Part model, mm, in its own coordinate system. A direction names the side the tool comes from. Round coordinates to 2 decimals unless told otherwise and drop trailing zeros. Loops run counter-clockwise (first coordinate to the right, second up) from the corner with the lowest first, then second, coordinate; pieces in that order, holes last. Notation, with made-up numbers: (2.25, 22) -> (53.25, 22) arc R14 ccw to (53.25, 36) -> close; hole circle Ø3 at (-27.75, 45). An arc over 180 degrees is marked (long way). Use a Markdown table: item, result. Add a question column.
Item 1: Which spindle directions (+Z, -Z, +X, -X, +Y, -Y) get a long thin tool onto all of the face, cutting with end or side? Do faces 1 (the face through (0, -12.5, 15)), 2 (the face through (-14.715, 0.231, 29.699)). Say none if no direction does.
Item 2: Cut at A-A, the plane y = 9. List the corners of the cut face in (x, z).
Item 3: Cut at C-C, the plane x = 0. List the corners of the cut face in (y, z), plus the area to 3 significant figures.
Item 4: Cut at B-B, the plane z = 15. List the corners of the cut face in (x, y).
Item 5: Two-plate mould, pull along X, no slides. Class faces 3 (the face through (-14.715, 17.199, 15.196)), 4 (the face through (1.5, 2.7, 19.77)), 5 (the face through (0.196, -17.215, 29.699)): pulls with the +X half, pulls with the -X half, needs draft (parallel to the pull), parting line crosses it, or undercut.
Item 6: Probe line 1 (X direction, y = 1, z = 15); line 2 (X direction, y = -6, z = 12); line 3 (Z direction, x = -0.75, y = 11). List the from-to ranges inside material, lowest first. Write a range as [from, to].
```python
from build123d import *

# Parameters (mm, degrees)
SKETCH1_W           = 30
SKETCH1_H           = 35
BOSS_EXTRUDE1_DEPTH = 30
SKETCH2_R           = 5
CUT_EXTRUDE1_DEPTH  = 30
FILLET2_R           = 1


with BuildPart() as part:
    # Sketch1 → Boss-Extrude1 (new body)
    with BuildSketch(Plane.XY):
        Rectangle(SKETCH1_W, SKETCH1_H)
    extrude(amount=BOSS_EXTRUDE1_DEPTH)

    # Sketch2 → Cut-Extrude1 (cut)
    with BuildSketch(Plane(origin=(0, 17.5, 0), x_dir=(1, 0, 0), z_dir=(0, 1, 0))):
        with Locations(Location((0, -15, 0), (0, 0, 270))):
            Circle(SKETCH2_R)
    extrude(amount=-CUT_EXTRUDE1_DEPTH, mode=Mode.SUBTRACT)

    # Fillet2
    fillet2_edges = [part.edges().sort_by_distance(p)[0] for p in [
        (-15, 0, 30),
        (0, -17.5, 30),
        (0, -12.5, 10),
        (0, 17.5, 10),
        (15, 0, 30),
        (0, -17.5, 0),
        (-15, 0, 0),
        (0, 17.5, 0),
        (15, 0, 0),
        (0, 17.5, 30),
        (15, -17.5, 15),
        (-15, -17.5, 15),
        (-15, 17.5, 15),
        (15, 17.5, 15),
    ]]
    fillet(fillet2_edges, radius=FILLET2_R)


solid = part.part
```
A:
| question | item | result |
|---|---|---|
| 1 | face 1 | +Y |
| 1 | face 2 | +Z, -X, +Y, -Y |
| 2 | outline | (-15, 1) arc R1 ccw to (-14, 0) -> (14, 0) arc R1 ccw to (15, 1) -> (15, 29) arc R1 ccw to (14, 30) -> (-14, 30) arc R1 ccw to (-15, 29) -> close; hole circle Ø10 at (0, 15) |
| 3 | outline | (-17.5, 1) arc R1 ccw to (-16.5, 0) -> (16.5, 0) arc R1 ccw to (17.5, 1) -> (17.5, 9) arc R1 ccw to (16.5, 10) -> (-11.5, 10) arc R1 cw to (-12.5, 11) -> (-12.5, 19) arc R1 cw to (-11.5, 20) -> (16.5, 20) arc R1 ccw to (17.5, 21) -> (17.5, 29) arc R1 ccw to (16.5, 30) -> (-16.5, 30) arc R1 ccw to (-17.5, 29) -> close |
| 3 | area | 749 mm^2 |
| 4 | outline | (-15, -16.5) arc R1 ccw to (-14, -17.5) -> (14, -17.5) arc R1 ccw to (15, -16.5) -> (15, 16.5) arc R1 ccw to (14, 17.5) -> (6, 17.5) arc R1 ccw to (5, 16.5) -> (5, -11.5) arc R1 cw to (4, -12.5) -> (-4, -12.5) arc R1 cw to (-5, -11.5) -> (-5, 16.5) arc R1 ccw to (-6, 17.5) -> (-14, 17.5) arc R1 ccw to (-15, 16.5) -> close |
| 5 | face 3 | pulls with the -X half |
| 5 | face 4 | undercut |
| 5 | face 5 | needs draft |
| 6 | line 1 | x = [-15, -5], [5, 15] |
| 6 | line 2 | x = [-15, -4], [4, 15] |
| 6 | line 3 | z = [0, 10.06], [19.94, 30] |
